Source: CAD feature listing. Evaluate the final solid. Frame: model axes, mm. Face numbers are marked on the shaded views. Give positions to 0.01 mm unless a question says otherwise; leave off trailing zeros. Write each loop counter-clockwise with the first axis right and the second up, starting at its lowest first coordinate (ties: lowest second). Pieces come first, ordered by that corner, then holes. Notation, with made-up numbers: M 63.25,-9.75 L 72.25,-9.75 A21 cw 72.25,6.25 Z; hole C 42,37.5 d2. An arc over 180 degrees is marked long. Return JSON: item names as keys, results as strings.
Autodesk Inventor part; units mm, degrees
ref_plane "YZ Plane" through (0, 0, 0) normal (1, 0, 0) x (0, 1, 0)
ref_plane "XZ Plane" through (0, 0, 0) normal (0, 1, 0) x (-1, 0, 0)
ref_plane "XY Plane" through (0, 0, 0) normal (0, 0, 1) x (1, 0, 0)
sketch "Skizze1" plane through (0, 0, 0) normal (0, 0, 1) x (1, 0, 0)
  circle A0 centre (0, 0) radius 27.5
  circle A1 centre (0, 0) radius 20
  line L0 (-6, 19.0788) -> (-6, 22.8)
  line L1 (-6, 22.8) -> (6, 22.8)
  line L2 (6, 22.8) -> (6, 19.0788)
  line L3 (0, -38.5) -> (0, 38.5) construction
  line L4 (-6, 20) -> (6, 20) construction
  line L5 (-11.3027, 16.5) -> (11.3027, 16.5)
  point P0 (0, 22.8)
  point P1 (0, 20)
  dimension "d0" = 2.8
  dimension "d1" = 12
  dimension "d2" = 40
  dimension "d3" = 55
  dimension "d9" = 3.5
extrude "Extrusion1" add sketch "Skizze1" along normal blind 11.8 contours A0 | L5 A1 | A1 L0 L1 L2 picked at (0.6759, 18.8958)
chamfer "Fase1" distance 0.5 angle 45 6 edges at (-27.5, 0, 11.8) (-27.5, 0, 0) (0, -20, 11.8) (0, 16.5, 11.8) (0, -20, 0) (0, 16.5, 0)
equation "\"d0\" = Nabennuttiefe_20"
equation "\"d1\" = Passfeder_width"
equation "\"d2\" = 2 * Shaft_CapstonPart_Dia"
equation "\"Shaft_CapstonPart_Length\" = 22.8"
properties part number "Capston_Distanzscheibe_10mm" material "Edelstahl"
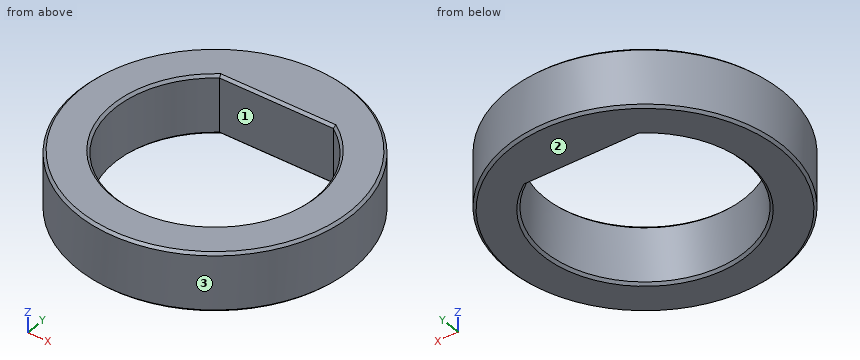
1) Cut plane C-C, the plane z = 2. Return the cut outline in (x, y).
Numbers:
{"outline": "C 0,0 d55; hole M -11.3,16.5 A20 ccw long 11.3,16.5 Z"}
2) Line query: line 1 (Y direction, x = 0, z = 6.75); line 2 (X direction, y = -4, z = 10.75); line 3 (X direction, y = -5, z = 6.5). Output: solid intervals per line, ascending. Write a range as [from, to].
Numbers:
{"line 1": "y = [-27.5, -20], [16.5, 27.5]", "line 2": "x = [-27.21, -19.6], [19.6, 27.21]", "line 3": "x = [-27.04, -19.36], [19.36, 27.04]"}
3) Draft query along Y for the marked faces 1, 2 and 3. Return one class per face: released by +Y, released by -Y, zero draft, split by the parting line, or undercut.
Numbers:
{"face 1": "undercut", "face 2": "zero draft", "face 3": "split by the parting line"}
4) Cut plane A-A, the plane y = 0. Return the cut outline in (x, z), then the cut area to 3 significant figures.
Numbers:
{"outline": "M -27.5,0.5 L -27,0 L -20.5,0 L -20,0.5 L -20,11.3 L -20.5,11.8 L -27,11.8 L -27.5,11.3 Z; M 20,0.5 L 20.5,0 L 27,0 L 27.5,0.5 L 27.5,11.3 L 27,11.8 L 20.5,11.8 L 20,11.3 Z", "area": "176 mm²"}
5) Cut plane B-B, the plane x = 0. Return the cut outline in (y, z), then the cut area to 3 significant figures.
Numbers:
{"outline": "M -27.5,0.5 L -27,0 L -20.5,0 L -20,0.5 L -20,11.3 L -20.5,11.8 L -27,11.8 L -27.5,11.3 Z; M 16.5,0.5 L 17,0 L 27,0 L 27.5,0.5 L 27.5,11.3 L 27,11.8 L 17,11.8 L 16.5,11.3 Z", "area": "217 mm²"}
6) Contact query for flat-ended pins moving along their axis: pin 1 Ø1 at (x, z) = (5, 7.5) entering from -Y; pin 2 Ø1.5 at (y, z) = (-4, 1.5) entering from +X; pin 3 Ø3 at (x, z) = (-3, 7) entering from -Y. Output: stop coordinate, or through.
Numbers:
{"pin 1": "stops at y = -27.13", "pin 2": "stops at x = 27.31", "pin 3": "stops at y = -27.46"}
